```python
from build123d import *

# Parameters (mm, degrees)
SALIENTE_EXTRUIR1_DEPTH = 1
CORTAR_EXTRUIR1_DEPTH   = 1
CROQUIS3_R              = 1.5
SALIENTE_EXTRUIR5_DEPTH = 20
CROQUIS4_R              = 1.5
SALIENTE_EXTRUIR6_DEPTH = 10
CROQUIS5_R              = 2.5
CORTAR_EXTRUIR2_DEPTH   = 1
CROQUIS7_R              = 1.5
SALIENTE_EXTRUIR7_DEPTH = 20


with BuildPart() as part:
    # Croquis1 → Saliente-Extruir1 (new body)
    with BuildSketch(Plane.XY):
        Polygon((-30, 279), (-382, 279), (-382, 260), (-412, 260), (-412, 2), (-382, 2), (-382, -17), (-30, -17), (-30, 2), (0, 2), (0, 260), (-30, 260), align=None)
        with BuildLine():
            Line((-371.5, 262.5), (-359.5, 262.5))
            ThreePointArc((-359.5, 262.5), (-357, 260), (-359.5, 257.5))
            Line((-359.5, 257.5), (-371.5, 257.5))
            ThreePointArc((-371.5, 257.5), (-374, 260), (-371.5, 262.5))
        make_face(mode=Mode.SUBTRACT)
        with BuildLine():
            Line((-371.5, -0.5), (-359.5, -0.5))
            ThreePointArc((-359.5, -0.5), (-357, 2), (-359.5, 4.5))
            Line((-359.5, 4.5), (-371.5, 4.5))
            ThreePointArc((-371.5, 4.5), (-374, 2), (-371.5, -0.5))
        make_face(mode=Mode.SUBTRACT)
    extrude(amount=SALIENTE_EXTRUIR1_DEPTH)

    # Croquis2 → Cortar-Extruir1 (cut)
    with BuildSketch(Plane.XY.offset(1)):
        with BuildLine():
            Line((-62.5, 257.5), (-74.5, 257.5))
            ThreePointArc((-74.5, 257.5), (-77, 260), (-74.5, 262.5))
            Line((-74.5, 262.5), (-62.5, 262.5))
            ThreePointArc((-62.5, 262.5), (-60, 260), (-62.5, 257.5))
        make_face()
        with BuildLine():
            Line((-62.5, 4.5), (-74.5, 4.5))
            ThreePointArc((-74.5, 4.5), (-77, 2), (-74.5, -0.5))
            Line((-74.5, -0.5), (-62.5, -0.5))
            ThreePointArc((-62.5, -0.5), (-60, 2), (-62.5, 4.5))
        make_face()
    extrude(amount=-CORTAR_EXTRUIR1_DEPTH, mode=Mode.SUBTRACT)

    # Croquis3 → Saliente-Extruir5 (add)
    with BuildSketch(Plane.XY.offset(1)):
        with Locations((-40, 212)):
            Circle(CROQUIS3_R)
        with Locations((-40, 50)):
            Circle(CROQUIS3_R)
        with Locations((-157, 50)):
            Circle(CROQUIS3_R)
        with Locations((-157, 212)):
            Circle(CROQUIS3_R)
    extrude(amount=SALIENTE_EXTRUIR5_DEPTH)

    # Croquis4 → Saliente-Extruir6 (add)
    with BuildSketch(Plane.XY.offset(1)):
        with Locations((-71.6, 197)):
            Circle(CROQUIS4_R)
        with Locations((-70, 63)):
            Circle(CROQUIS4_R)
        with Locations((-137, 63)):
            Circle(CROQUIS4_R)
        with Locations((-145.6, 197)):
            Circle(CROQUIS4_R)
    extrude(amount=SALIENTE_EXTRUIR6_DEPTH)

    # Croquis5 → Cortar-Extruir2 (cut)
    with BuildSketch(Plane.XY.offset(1)):
        with Locations((-332, 216)):
            Circle(CROQUIS5_R)
        with Locations((-332, 46)):
            Circle(CROQUIS5_R)
        with Locations((-314, 216)):
            Circle(CROQUIS5_R)
        with Locations((-314, 46)):
            Circle(CROQUIS5_R)
        with Locations((-270, 46)):
            Circle(CROQUIS5_R)
        with Locations((-252, 46)):
            Circle(CROQUIS5_R)
        with Locations((-270, 216)):
            Circle(CROQUIS5_R)
        with Locations((-252, 216)):
            Circle(CROQUIS5_R)
    extrude(amount=-CORTAR_EXTRUIR2_DEPTH, mode=Mode.SUBTRACT)

    # Croquis7 → Saliente-Extruir7 (add)
    with BuildSketch(Plane.XY.offset(1)):
        with Locations((-124.5, 266)):
            Circle(CROQUIS7_R)
        with Locations((-124.5, 254)):
            Circle(CROQUIS7_R)
    extrude(amount=SALIENTE_EXTRUIR7_DEPTH)


solid = part.part
```
The listing builds one solid part. Answer for the finished solid, in the listing's coordinates (mm). Coordinates: 2 decimals unless noted, no trailing zeros. Loops run counter-clockwise (first coordinate to the right, second up) from the corner with the lowest first, then second, coordinate; pieces in that order, holes last. Notation, with made-up numbers: (77.5, 40.5) -> (105.5, 40.5) arc R21 cw to (105.5, 67.5) -> close; hole circle Ø10 at (-19, -19). An arc over 180 degrees is marked (long way). Return JSON: item names as keys, results as strings. Group by question number.
(1) Find the intervals of material crossed by probe 1 along Y at (x, z) = (-270, 0.8); probe 2 along X at (y, z) = (216, 0.5); probe 3 along Z at (x, y) = (-132.5, 72), in increasing order. Write a range as from..to.
(2) Given pin 1 Ø0.5 at (x, z) = (-404, 0.5) entering from -Y; pin 2 Ø6.5 at (x, y) = (-332, 46) entering from -Z; pin 3 Ø0.8 at (y, z) = (-9.5, 0.5) entering from -X; pin 4 Ø1.5 at (x, y) = (-137.5, 62.5) entering from +Z, each flat-ended and moving along its own axis, determine where each tip first touches the part or whether it passes through.
(3) A cutting plane is placed at C-C on x = -215. Write down the section's boundary in (y, z), and give its area (3 significant figures).
(4) A cutting plane is placed at B-B on y = 90. Write down the section's boundary in (x, z), and give its area (3 significant figures).
(5) A cutting plane is placed at A-A on z = 17.5. Write down the section's boundary in (x, y).
The answers:
{
 "1": {"probe 1": "y = -17..43.5, 48.5..213.5, 218.5..279", "probe 2": "x = -412..-334.5, -329.5..-316.5, -311.5..-272.5, -267.5..-254.5, -249.5..0", "probe 3": "z = 0..1"},
 "2": {"pin 1": "stops at y = 2", "pin 2": "stops at z = 0", "pin 3": "stops at x = -382", "pin 4": "stops at z = 11"},
 "3": {"outline": "(-17, 0) -> (279, 0) -> (279, 1) -> (-17, 1) -> close", "area": "296 mm^2"},
 "4": {"outline": "(-412, 0) -> (0, 0) -> (0, 1) -> (-412, 1) -> close", "area": "412 mm^2"},
 "5": {"outline": "circle Ø3 at (-157, 50); circle Ø3 at (-157, 212); circle Ø3 at (-124.5, 254); circle Ø3 at (-124.5, 266); circle Ø3 at (-40, 50); circle Ø3 at (-40, 212)"}
}
